Read the model definition and answer for the solid it produces. Units are mm, in the model's axes. A direction names the side the tool comes from. Give positions to 0.01 mm unless a question says otherwise; leave off trailing zeros. Loops run counter-clockwise (first coordinate to the right, second up) from the corner with the lowest first, then second, coordinate; pieces in that order, holes last. Notation, with made-up numbers: (-33, 64) - (7, 64) arc R27 ccw to (7, 81) - close; hole circle Ø7 at (86.25, 32). An arc over 180 degrees is marked (long way). Put each result on its own line as item: value. Start each with the question number.
1. A cutting plane is placed at B-B, the plane z = 1.5. Count the separate pieces of the cut face and the enclosed holes in it, plus the area to 3 significant figures.
2. For faces 1 (the flat face through (7.952, 5, 1.5)), 2 (the flat face through (2.5, 4.034, 1.5)), 3 (the flat face through (9.917, 5, 1.5)), determine the directions among +Z, -Z, +X, -X, +Y, -Y from which every point of the face is accessible in a straight line to the end or side of a thin tool.
3. Consider L1, parallel to Y at x = 28.5, z = 1.7; L2, parallel to Y at x = 17, z = 1.6; L3, parallel to Z at x = 13, y = 6. Determine where each line is inside the solid, lowest interval first. Write a range as from..to.
4. For a pull along X with two mould halves and no side action, classify faces 4 (the flat face through (23, 9.007, 1.5)), 5 (the flat face through (5, 2.992, 1.5)) as released by +X, released by -X, zero draft, split by the parting line, or undercut.
5. A cutting plane is placed at A-A, the plane x = 4.5. Determine the outline of the cut face in (y, z), plus the area to 3 significant figures.
6. A cutting plane is placed at C-C, the plane y = 3.5. Determine the outline of the cut face in (x, z).
7. Given pin 1 Ø0.8 at (x, z) = (14.5, 1.5) entering from +Y; pin 2 Ø0.5 at (x, z) = (26.5, 1.5) entering from -Y, each flat-ended and moving along its own axis, determine where each tip first touches the part or whether it passes through.
8. A cutting plane is placed at D-D, the plane x = 11.5. Determine the outline of the cut face in (y, z).
```python
from build123d import *

# Parameters (mm, degrees)
SKETCH_W       = 30.047779
SKETCH_H       = 10.025875
PAD_DEPTH      = 1
SKETCH001_W    = 1.995144
SKETCH001_H    = 2.024921
SKETCH001_W_2  = 1.965365
SKETCH001_H_2  = 1.965365
SKETCH001_W_3  = 1.965363
SKETCH001_H_3  = 1.995143
SKETCH001_W_4  = 1.995143
SKETCH001_W_5  = 2.024922
SKETCH001_W_6  = 1.965367
SKETCH001_W_7  = 1.995147
SKETCH001_W_8  = 0.982683
SKETCH001_W_9  = 1.012457
SKETCH001_W_10 = 0.952904
SKETCH001_H_4  = 2.024922
SKETCH001_W_11 = 1.012463
SKETCH001_H_5  = 1.965366
SKETCH001_W_12 = 0.952906
SKETCH001_W_13 = 2.977825
SKETCH001_W_14 = 1.965366
SKETCH001_H_6  = 1.995144
SKETCH001_W_15 = 2.024921
SKETCH001_W_16 = 1.965361
SKETCH001_W_17 = 1.99514
SKETCH001_W_18 = 1.965362
SKETCH001_W_19 = 2.024923
SKETCH001_H_7  = 1.965364
SKETCH001_W_20 = 1.995142
PAD001_DEPTH   = 1


with BuildPart() as part:
    # Sketch → Pad (new body)
    with BuildSketch(Plane.XY):
        with Locations((15.023889, 5.012937)):
            Rectangle(SKETCH_W, SKETCH_H)
    extrude(amount=PAD_DEPTH)

    # Sketch001 (on Face6 of Pad) → Pad001 (join)
    with BuildSketch(Plane.XY.offset(1)):
        with Locations((2.041063, 2.009386)):
            Rectangle(SKETCH001_W, SKETCH001_H)
        with Locations((5.003999, 2.009385)):
            Rectangle(SKETCH001_W_2, SKETCH001_H_2)
        with Locations((7.981825, 1.964719)):
            Rectangle(SKETCH001_W_3, SKETCH001_H_3)
        with Locations((11.004319, 1.979607)):
            Rectangle(SKETCH001_W_4, SKETCH001_H)
        with Locations((14.026814, 2.024274)):
            Rectangle(SKETCH001_W_5, SKETCH001_H_3)
        with Locations((17.004638, 2.024274)):
            Rectangle(SKETCH001_W_6, SKETCH001_H_3)
        with Locations((19.997352, 1.979607)):
            Rectangle(SKETCH001_W_7, SKETCH001_H_2)
        with Locations((23.019848, 1.979607)):
            Rectangle(SKETCH001_W_5, SKETCH001_H_2)
        with Locations((28.484158, 1.964719)):
            Rectangle(SKETCH001_W_8, SKETCH001_H_3)
        with Locations((26.53368, 2.009386)):
            Rectangle(SKETCH001_W_9, SKETCH001_H)
        with Locations((26.503904, 5.016991)):
            Rectangle(SKETCH001_W_10, SKETCH001_H_2)
        with Locations((28.484158, 5.01699)):
            Rectangle(SKETCH001_W_8, SKETCH001_H_4)
        with Locations((26.444347, 7.965038)):
            Rectangle(SKETCH001_W_11, SKETCH001_H_5)
        with Locations((28.499047, 7.994816)):
            Rectangle(SKETCH001_W_12, SKETCH001_H_4)
        with Locations((2.502625, 5.03188)):
            Rectangle(SKETCH001_W_13, SKETCH001_H_3)
        with Locations((2.026174, 7.965037)):
            Rectangle(SKETCH001_W_14, SKETCH001_H)
        with Locations((4.98911, 8.039484)):
            Rectangle(SKETCH001_W, SKETCH001_H_6)
        with Locations((6.04624, 5.046768)):
            Rectangle(SKETCH001_W_15, SKETCH001_H_2)
        with Locations((8.934731, 5.01699)):
            Rectangle(SKETCH001_W_2, SKETCH001_H_4)
        with Locations((11.972112, 5.016991)):
            Rectangle(SKETCH001_W_15, SKETCH001_H_2)
        with Locations((14.94994, 4.987212)):
            Rectangle(SKETCH001_W_14, SKETCH001_H_5)
        with Locations((18.017098, 5.01699)):
            Rectangle(SKETCH001_W_16, SKETCH001_H_4)
        with Locations((21.009815, 5.002101)):
            Rectangle(SKETCH001_W, SKETCH001_H_6)
        with Locations((24.047197, 5.01699)):
            Rectangle(SKETCH001_W_17, SKETCH001_H_4)
        with Locations((8.026494, 8.009705)):
            Rectangle(SKETCH001_W, SKETCH001_H_3)
        with Locations((11.034097, 7.979926)):
            Rectangle(SKETCH001_W_4, SKETCH001_H_3)
        with Locations((13.997034, 7.965037)):
            Rectangle(SKETCH001_W_18, SKETCH001_H)
        with Locations((17.019527, 8.054373)):
            Rectangle(SKETCH001_W, SKETCH001_H_5)
        with Locations((20.01224, 7.994816)):
            Rectangle(SKETCH001_W_19, SKETCH001_H_7)
        with Locations((23.004958, 8.009705)):
            Rectangle(SKETCH001_W_20, SKETCH001_H_3)
    extrude(amount=PAD001_DEPTH)


solid = part.part
```
Return value:
1. separate pieces: 30
1. enclosed holes: 0
1. area: 109 mm2
2. face 1: +Z
2. face 2: +Z, -X
2. face 3: +Z, +Y, -Y
3. L1: y = 0.97..2.96, 4..6.03, 6.98..9.01
3. L2: y = 1.03..3.02, 7.07..9.04
3. L3: z = 0..1
4. face 4: zero draft
4. face 5: undercut
5. outline: (0, 0) - (10.03, 0) - (10.03, 1) - (9.04, 1) - (9.04, 2) - (7.04, 2) - (7.04, 1) - (2.99, 1) - (2.99, 2) - (1.03, 2) - (1.03, 1) - (0, 1) - close
5. area: 14.0 mm2
6. outline: (0, 0) - (30.05, 0) - (30.05, 1) - (0, 1) - close
7. pin 1: stops at y = 8.98
7. pin 2: stops at y = 1
8. outline: (0, 0) - (10.03, 0) - (10.03, 1) - (8.98, 1) - (8.98, 2) - (6.98, 2) - (6.98, 1) - (6, 1) - (6, 2) - (4.03, 2) - (4.03, 1) - (2.99, 1) - (2.99, 2) - (0.97, 2) - (0.97, 1) - (0, 1) - close
